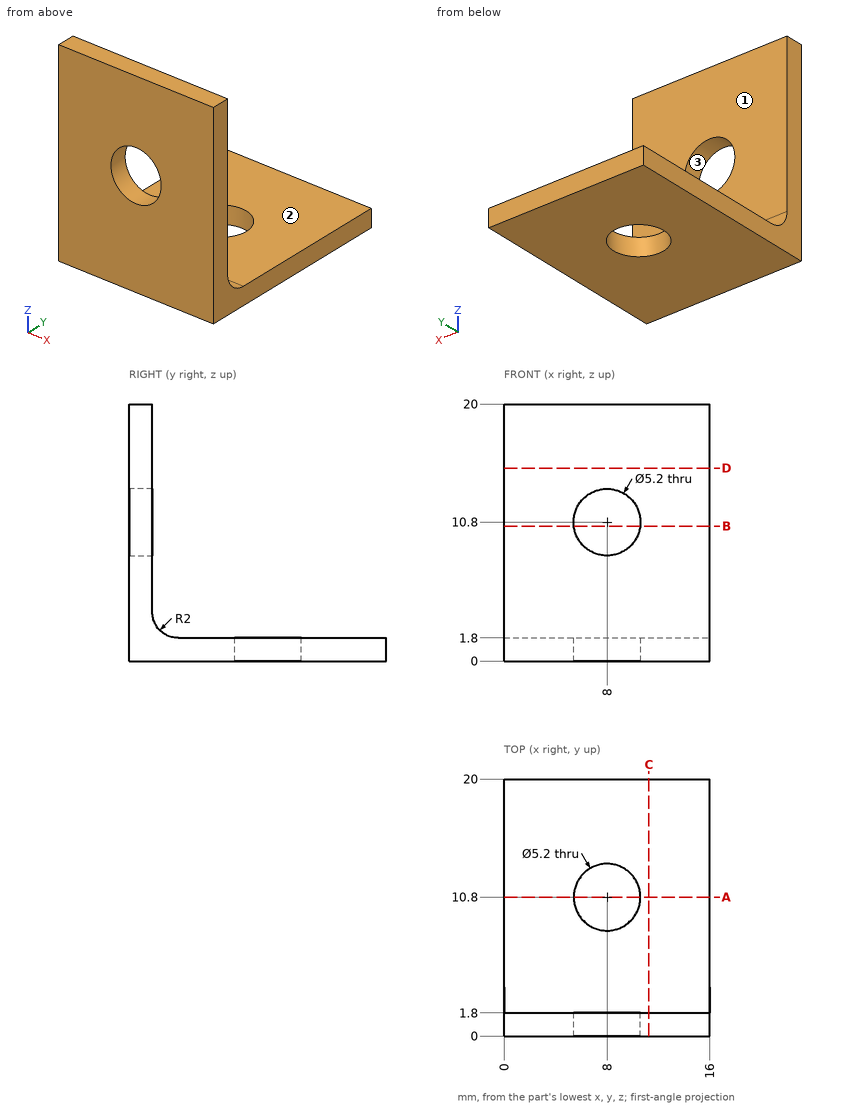
Source: three-view drawing plus pictorial views. Frame: mm from the lowest corner of the part. Give positions to 0.01 mm unless a question says otherwise; leave off trailing zeros. Write each loop counter-clockwise with the first axis right and the second up, starting at its lowest first coordinate (ties: lowest second). Pieces come first, ordered by that corner, then holes.
(1) Cut plane B-B, the plane z = 10.5. Return loops of the section in (x, y), then the cut area to 3 significant figures.
(2) Cut plane A-A, the plane y = 10.8. Return loops of the section in (x, z), then the cut area to 3 significant figures.
(3) Ray query, line 1 (X direction, y = 0.8, z = 10.8); line 2 (Y direction, x = 8, z = 0.65); line 3 (Y direction, x = 5.5, z = 17). Return the intervals inside material, ascending.
(4) First-contact query: P1, Ø6, axis at x = 11.5, y = 3, coming from the +Z side; P2, Ø8, axis at x = 10.5, y = 11, coming from the +Z side; P3, Ø3, axis at x = 4, z = 15, coming from the +Y side. Flat tips, straight axial feed; report the tip coordinate or a pass-through.
(5) Cut plane D-D, the plane z = 15. Return loops of the section in (x, y).
(6) Cut plane C-C, the plane x = 11.25. Return loops of the section in (y, z).
(7) Mould query, pull axis Z, two halves, no side actions, for the marked faces 1, 2 and 3. Classes: released by +Z, released by -Z, zero draft, split by the parting line, or undercut.
Values follow:
1. outline: (0, 0) - (5.42, 0) - (5.42, 1.8) - (0, 1.8) - close; (10.58, 0) - (16, 0) - (16, 1.8) - (10.58, 1.8) - close
1. area: 19.5 mm2
2. outline: (0, 0) - (5.4, 0) - (5.4, 1.8) - (0, 1.8) - close; (10.6, 0) - (16, 0) - (16, 1.8) - (10.6, 1.8) - close
2. area: 19.4 mm2
3. line 1: x = 0 to 5.4, 10.6 to 16
3. line 2: y = 0 to 8.2, 13.4 to 20
3. line 3: y = 0 to 1.8
4. P1: stops at z = 20
4. P2: stops at z = 1.8
4. P3: stops at y = 1.8
5. outline: (0, 0) - (16, 0) - (16, 1.8) - (0, 1.8) - close
6. outline: (0, 0) - (20, 0) - (20, 1.8) - (3.8, 1.8) arc R2 cw to (1.8, 3.8) - (1.8, 20) - (0, 20) - close
7. face 1: zero draft
7. face 2: released by +Z
7. face 3: undercut
